Geometry check sheet. Reference: the model listing, model coordinates, mm. Face numbers are marked on the shaded views. A direction names the side the tool comes from. Round coordinates to 2 decimals unless told otherwise and drop trailing zeros. Write each loop counter-clockwise with the first axis right and the second up, starting at its lowest first coordinate (ties: lowest second). Pieces come first, ordered by that corner, then holes. Notation, with made-up numbers: (60, 4) - (79, 4) arc R8 cw to (79, 9) - close; hole circle Ø6 at (-26, 14). An arc over 180 degrees is marked (long way). Return JSON: item names as keys, results as strings.
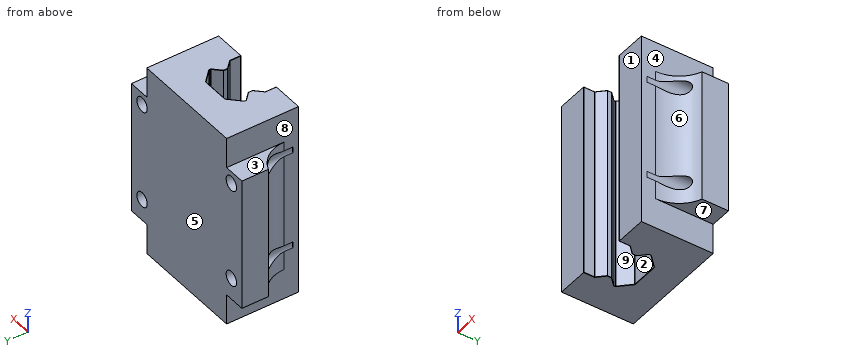
```python
from build123d import *

# Parameters (mm, degrees)
SKETCH_4_W          = 34
SKETCH_4_H          = 21.7
EXTRUDE_2_DEPTH     = 58.6
CUT_EXTRUDE_1_DEPTH = 58.6
FILLET_1_R          = 0.1
EXTRUDE_4_DEPTH     = 6.5
EXTRUDE_5_DEPTH     = 6.5
FILLET_3_R          = 10
FILLET_4_R          = 10
SKETCH_11_R         = 2.2
CUT_EXTRUDE_2_DEPTH = 20


with BuildPart() as part:
    # Эскиз4 → Бобышка-Вытянуть2 (new body)
    with BuildSketch(Plane.XY):
        Rectangle(SKETCH_4_W, SKETCH_4_H)
    extrude(amount=EXTRUDE_2_DEPTH)

    # Эскиз5 → Вырез-Вытянуть1 (cut)
    with BuildSketch(Plane(origin=(0, 0, 0), x_dir=(-1, 0, 0), z_dir=(0, 0, -1))):
        Polygon((0, -10.85), (7.5, -10.85), (7.5, -7.55), (5.26, -5.31), (5.26, -3.989299906), (7.5, -1.749299906), (7.5, -1.249299906), (4.100700094, 2.15), (-4.100700094, 2.15), (-7.5, -1.249299906), (-7.5, -1.749299906), (-5.26, -3.989299906), (-5.26, -5.31), (-7.5, -7.55), (-7.5, -10.85), align=None)
    extrude(amount=-CUT_EXTRUDE_1_DEPTH, mode=Mode.SUBTRACT)

    # Скругление1
    fillet_1_edges = [part.edges().sort_by_distance(p)[0] for p in [
        (7.5, -9.2, 58.6),
        (7.5, -10.85, 29.3),
        (6.38, -6.43, 58.6),
        (7.5, -7.55, 29.3),
        (5.26, -4.649649953, 58.6),
        (5.26, -5.31, 29.3),
        (6.38, -2.869299906, 58.6),
        (5.26, -3.989299906, 29.3),
        (7.5, -1.499299906, 58.6),
        (7.5, -1.749299906, 29.3),
        (5.800350047, 0.450350047, 58.6),
        (7.5, -1.249299906, 29.3),
        (0, 2.15, 58.6),
        (4.100700094, 2.15, 29.3),
        (-5.800350047, 0.450350047, 58.6),
        (-4.100700094, 2.15, 29.3),
        (-7.5, -1.499299906, 58.6),
        (-7.5, -1.249299906, 29.3),
        (-6.38, -2.869299906, 58.6),
        (-7.5, -1.749299906, 29.3),
        (-5.26, -4.649649953, 58.6),
        (-5.26, -3.989299906, 29.3),
        (-6.38, -6.43, 58.6),
        (-5.26, -5.31, 29.3),
        (-7.5, -9.2, 58.6),
        (-7.5, -7.55, 29.3),
        (-7.5, -10.85, 29.3),
        (7.5, -9.2, 0),
        (-7.5, -9.2, 0),
        (-6.38, -6.43, 0),
        (-5.26, -4.649649953, 0),
        (-6.38, -2.869299906, 0),
        (-7.5, -1.499299906, 0),
        (-5.800350047, 0.450350047, 0),
        (0, 2.15, 0),
        (5.800350047, 0.450350047, 0),
        (7.5, -1.499299906, 0),
        (6.38, -2.869299906, 0),
        (5.26, -4.649649953, 0),
        (6.38, -6.43, 0),
    ]]
    fillet(fillet_1_edges, radius=FILLET_1_R)

    # Эскиз9 → Бобышка-Вытянуть4 (add)
    with BuildSketch(Plane(origin=(17, 0, 0), x_dir=(0, 0, -1), z_dir=(1, 0, 0))):
        Polygon((-29.3, 10.85), (-9.2, 10.85), (-9.2, 2.85), (-49.4, 2.85), (-49.4, 10.85), align=None)
    extrude(amount=EXTRUDE_4_DEPTH)

    # Эскиз10 → Бобышка-Вытянуть5 (add)
    with BuildSketch(Plane.ZY.offset(17)):
        Polygon((29.3, 10.85), (49.4, 10.85), (49.4, 2.85), (9.2, 2.85), (9.2, 10.85), align=None)
    extrude(amount=EXTRUDE_5_DEPTH)

    # Скругление3
    # the kernel refuses this fillet: 10 mm, written as the material it adds along each edge
    with BuildSketch(Plane(origin=(-17, 2.85, 49.4), x_dir=(0, -1, 0), z_dir=(0, 0, -1))) as fillet_3_piece_1:
        with BuildLine():
            CenterArc((9.367496998, 10), FILLET_3_R, 200.487315115, 69.512684885)
            Line((0, 6.5), (-0.18734994, 6.43))
            ThreePointArc((-0.18734994, 6.43), (-0.2, 3.25), (-0.2, 0))
            Line((-0.2, 0), (0, -0.2))
            Line((0, -0.2), (9.367496998, -0.2))
            Line((9.367496998, -0.2), (9.367496998, 0))
        make_face()
    extrude(amount=40.2)

    # Скругление4
    # the kernel refuses this fillet: 10 mm, written as the material it adds along each edge
    with BuildSketch(Plane(origin=(17, 2.85, 9.2), x_dir=(1, 0, 0), z_dir=(0, 0, 1))) as fillet_4_piece_1:
        with BuildLine():
            CenterArc((10, -9.367496998), FILLET_4_R, 110.487315115, 69.512684885)
            Line((0, -9.367496998), (-0.2, -9.367496998))
            Line((-0.2, -9.367496998), (-0.2, 0))
            Line((-0.2, 0), (0, 0.2))
            ThreePointArc((0, 0.2), (3.25, 0.2), (6.43, 0.18734994))
            Line((6.43, 0.18734994), (6.5, 0))
        make_face()
    extrude(amount=40.2)

    # Эскиз11 → Вырез-Вытянуть2 (cut)
    with BuildSketch(Plane(origin=(0, 10.85, 0), x_dir=(1, 0, 0), z_dir=(0, 1, 0))):
        with Locations(Location((-19, -15.723228877, 0), (0, 0, 270))):
            Circle(SKETCH_11_R)
        with Locations(Location((19, -15.723228877, 0), (0, 0, 270))):
            Circle(SKETCH_11_R)
        with Locations(Location((-19, -45.723228877, 0), (0, 0, 270))):
            Circle(SKETCH_11_R)
        with Locations(Location((19, -45.723228877, 0), (0, 0, 270))):
            Circle(SKETCH_11_R)
    extrude(amount=-CUT_EXTRUDE_2_DEPTH, mode=Mode.SUBTRACT)


solid = part.part
```
(1) Access from +Z, -Z, +X, -X, +Y, -Y to the whole of each face (thin tool, end or side, straight path). Record for the marked faces 1, 2, 3, 4 and 5.
Response values:
{"face 1": "+Z, -Z, +X, -X, -Y", "face 2": "+Z, -Z, -Y", "face 3": "+Z, -X, +Y, -Y", "face 4": "+X, -Y", "face 5": "+Z, -Z, +X, -X, +Y"}
(2) Release check for a two-part mould opening along X. For the marked faces 6, 7, 8 and 9 record: pulls with the +X half, pulls with the -X half, needs draft (parallel to the pull), parting line crosses it, or undercut.
Response values:
{"face 6": "pulls with the +X half", "face 7": "needs draft", "face 8": "pulls with the -X half", "face 9": "undercut"}
(3) Gauge pin test, flat ends, axial feed: pin 1 (5 mm diameter, centred on y = 8, z = 7, fed in from -X); pin 2 (2 mm diameter, centred on x = -19.5, y = 2.5, fed in from +Z); pin 3 (3 mm diameter, centred on x = -21.5, y = 1, fed in from -Z); pin 4 (3.5 mm diameter, centred on x = 19, z = 45.72, fed in from +Y). Record the tip position at first contact, or that the pin passes through.
Response values:
{"pin 1": "stops at x = -23.5", "pin 2": "stops at z = 49.4", "pin 3": "stops at z = 9.2", "pin 4": "passes through"}
(4) Section check C-C, the plane x = 2. Enter the section's corners in (y, z), plus the area to 3 significant figures.
Response values:
{"outline": "(2.15, 0.1) arc R0.1 ccw to (2.25, 0) - (10.85, 0) - (10.85, 58.6) - (2.25, 58.6) arc R0.1 ccw to (2.15, 58.5) - close", "area": "510 mm^2"}
(5) Section check A-A, the plane x = 19. Enter the section's corners in (y, z).
Response values:
{"outline": "(-0.52, 9.2) - (10.85, 9.2) - (10.85, 13.52) - (-0.52, 13.52) - close; (-0.52, 17.92) - (10.85, 17.92) - (10.85, 43.52) - (-0.52, 43.52) - close; (-0.52, 47.92) - (10.85, 47.92) - (10.85, 49.4) - (-0.52, 49.4) - close"}
(6) Material ranges on line 1 along Z through (x, y) = (19, 3.25); line 2 along X through (y, z) = (-7.75, 40); line 3 along X through (y, z) = (8.5, 14), recorded low to high. Write a range as [from, to].
Response values:
{"line 1": "z = [9.2, 13.52], [17.92, 43.52], [47.92, 49.4]", "line 2": "x = [-17, -7.5], [7.5, 17]", "line 3": "x = [-23.5, -20.37], [-17.63, 17.63], [20.37, 23.5]"}
